Here's the drawing with two shaded views (mm, measured from the low corner). I have some questions. A direction names the side the tool comes from. Coordinates: 2 decimals unless noted, no trailing zeros. Write each loop counter-clockwise with the first axis right and the second up, starting at its lowest first coordinate (ties: lowest second). Pieces come first, ordered by that corner, then holes. Notation, with made-up numbers: M 70.5,-38.75 L 125.5,-38.75 A15 cw 125.5,-17.75 Z; hole C -10.75,73 d7. An arc over 180 degrees is marked long. Answer as CSV lines item,"result". Start each with the question number.
Item 1: Suppose I cut it at D-D, the plane z = 3.5. Write out the boundary of the cut face in (x, y).
Item 2: I'm going to push flat-ended pins straight in: P1, Ø3.5, axis at x = 10, z = 10, coming from the -Y side; P2, Ø2, axis at x = 9.5, z = 4, coming from the +Y side. Where does each tip first touch, or does it pass through?
Item 3: We'd pull the mould along Z, two halves only. Please class the marked faces 3, 4 and 5: +Z half, -Z half, draft (parallel to the pull), parting line (faces both ways), or undercut.
Item 4: Suppose I cut it at B-B, the plane x = 2.25. Write out the boundary of the cut face in (y, z), and give its area (3 significant figures).
Item 5: If I drill on line 1 along X through (y, z) = (1.55, 10); line 2 along Y through (x, z) = (17, 5.5), over which ranges is the centre line in solid material (lowest first)? Write a range as [from, to].
Item 6: Suppose I cut it at C-C, the plane y = 1. Write out the boundary of the cut face in (x, z), and give its area (3 significant figures).
Item 7: On a 3-axis mill with a long thin cutter (end or side, diameter ignored), from which of +Z, -Z, +X, -X, +Y, -Y can I reach the whole of each face in a straight line? I mean the marked faces 1 and 2. Say none if no direction works.
Item 8: Suppose I cut it at A-A, the plane z = 10. Write out the boundary of the cut face in (x, y).
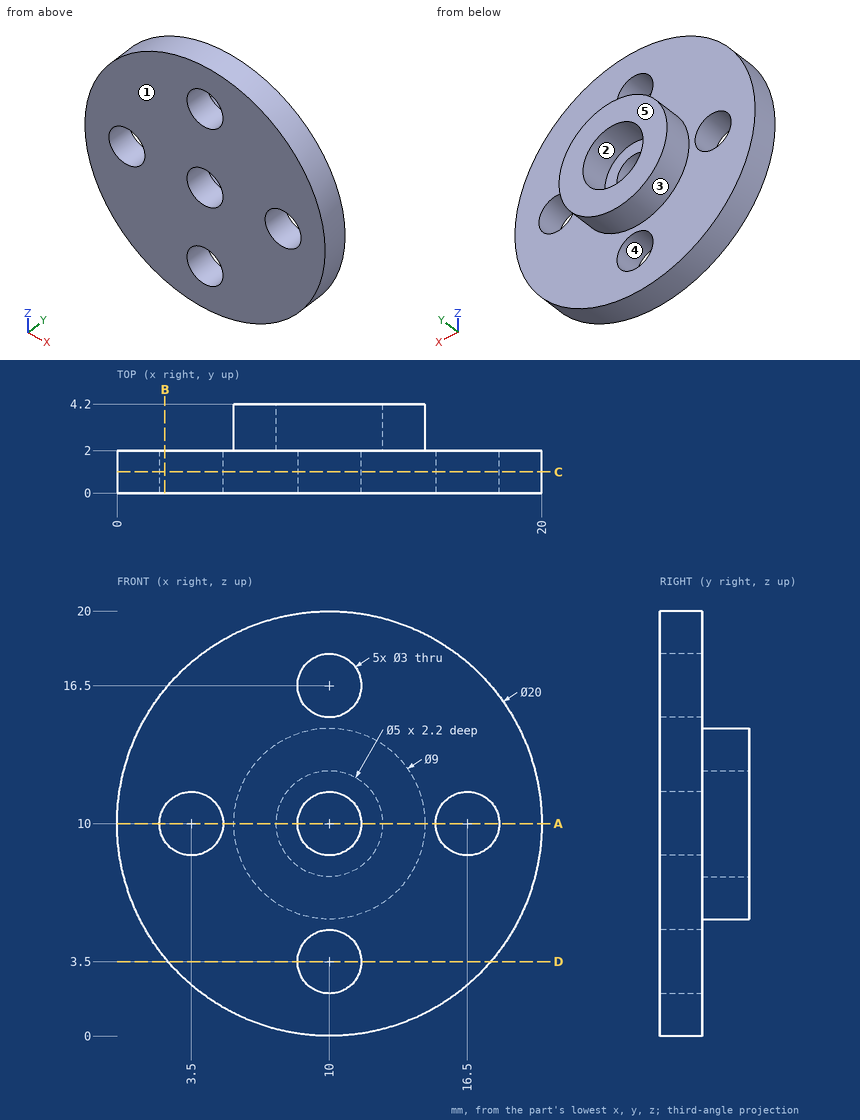
Ans:
1,outline,"M 2.4,0 L 8.5,0 L 8.5,2 L 2.4,2 Z; M 11.5,0 L 17.6,0 L 17.6,2 L 11.5,2 Z"
2,P1,"stops at y = 0"
2,P2,"stops at y = 2"
3,face 3,"parting line"
3,face 4,"undercut"
3,face 5,"draft"
4,outline,"M 0,3.68 L 2,3.68 L 2,9.17 L 0,9.17 Z; M 0,10.83 L 2,10.83 L 2,16.32 L 0,16.32 Z"
4,area,"22.0 mm^2"
5,line 1,"x = [0, 2], [5, 8.5], [11.5, 15], [18, 20]"
5,line 2,"y = [0, 2]"
6,outline,"C 10,10 d20; hole C 3.5,10 d3; hole C 10,3.5 d3; hole C 10,10 d3; hole C 10,16.5 d3; hole C 16.5,10 d3"
6,area,"279 mm^2"
7,face 1,"+Z, -Z, +X, -X, -Y"
7,face 2,"+Y"
8,outline,"M 0,0 L 2,0 L 2,2 L 0,2 Z; M 5,0 L 8.5,0 L 8.5,2 L 7.5,2 L 7.5,4.2 L 5.5,4.2 L 5.5,2 L 5,2 Z; M 11.5,0 L 15,0 L 15,2 L 14.5,2 L 14.5,4.2 L 12.5,4.2 L 12.5,2 L 11.5,2 Z; M 18,0 L 20,0 L 20,2 L 18,2 Z"
